Check sheet for the modelled part. Datum: model origin and axes. Units: mm. A direction names the side the tool comes from. Round coordinates to 2 decimals unless told otherwise and drop trailing zeros. Write each loop counter-clockwise with the first axis right and the second up, starting at its lowest first coordinate (ties: lowest second). Pieces come first, ordered by that corner, then holes. Notation, with made-up numbers: (80.25, 20.25) -> (102.25, 20.25) arc R24 ccw to (102.25, 57.25) -> close; hole circle Ø1 at (83, -35). An arc over 180 degrees is marked (long way). Write item = value, one per line.
from build123d import *

# Parameters (mm, degrees)
SKETCH11_R              = 1.7859375
CUT_EXTRUDE1_DEPTH      = 6.588
CUT_EXTRUDE1_DEPTH_BACK = 6.588


with BuildPart() as part:
    # Sketch10 → Revolve1 (revolve)
    with BuildSketch(Plane(origin=(0, 0, 0), x_dir=(0, 0, -1), z_dir=(1, 0, 0))):
        Polygon((6.35, 3.571875), (6.35, 0), (-8.89, 0), (-8.89, 5.08), (-8.382, 5.588), (-6.35, 5.588), (-6.35, 3.96875), (5.953125, 3.96875), align=None)
    revolve(axis=Axis((0, 0, 6.35), (0, 0, -1)))

    # Sketch11 → Cut-Extrude1 (cut, two sides)
    with BuildSketch(Plane(origin=(0, 0, 0), x_dir=(0, 0, -1), z_dir=(1, 0, 0))) as cut_extrude1_sk:
        with Locations((1.7859375, 0)):
            Circle(SKETCH11_R)
    extrude(amount=CUT_EXTRUDE1_DEPTH, mode=Mode.SUBTRACT)
    extrude(cut_extrude1_sk.sketch, amount=-CUT_EXTRUDE1_DEPTH_BACK, mode=Mode.SUBTRACT)


solid = part.part
(1) Sectioned sample at A-A on z = 4.25. Enter the section's corners in (x, y).
Worked answers:
outline = circle Ø7.94 at (0, 0)
(2) Access from +Z, -Z, +X, -X, +Y, -Y to the whole of each face (thin tool, end or side, straight path). Record for faces 3 (the flat face through (0, 0, 8.89)), 4 (the flat face through (4, 1, 6.35)).
Worked answers:
face_3 = +Z, +X, -X, +Y, -Y
face_4 = -Z
(3) Material ranges on L1, parallel to Z at x = 1.75, y = 0; L2, parallel to Z at x = 4, y = -2.25; L3, parallel to Y at x = -3, z = -1.75, recorded low to high. Write a range as [from, to].
Worked answers:
L1 = [-6.35, -3.57], [0, 8.89]
L2 = [6.35, 8.89]
L3 = [-2.6, -1.79], [1.79, 2.6]
(4) Release check for a two-part mould opening along X. For faces 1 (the flat face through (0, 0, -6.35)), 2 (the cylindrical face through (-1.52, 3.666, 0.112)) record: pulls with the +X half, pulls with the -X half, needs draft (parallel to the pull), parting line crosses it, or undercut.
Worked answers:
face_1 = needs draft
face_2 = parting line crosses it
(5) Go/stop test with flat-tipped pins: P1, Ø2, axis at y = -4, z = 7, coming from the +X side; P2, Ø1.5, axis at y = 1.5, z = 0.5, coming from the -X side; P3, Ø2, axis at y = 0, z = -1.79, coming from the +X side; P4, Ø1, axis at x = 2, z = -2.5, coming from the -Y side. Record where each tip stops, or that it passes through.
Worked answers:
P1 = 4.71
P2 = -3.9
P3 = through
P4 = -3.67
